Can you work these out from the model? Positions are in its coordinate system, mm. A direction names the side the tool comes from. Give positions to 0.01 mm unless a question says otherwise; leave off trailing zeros. Loops run counter-clockwise (first coordinate to the right, second up) from the corner with the lowest first, then second, coordinate; pieces in that order, holes last. Notation, with made-up numbers: (7, 81.25) - (46, 81.25) arc R15 cw to (46, 92.25) - close; hole circle Ø3 at (46.25, 3). An arc over 180 degrees is marked (long way). Answer as a JSON object with one key per item and string values. Group by question number.
Item 1: Which directions (+Z, -Z, +X, -X, +Y, -Y) give clear straight access to the entire face, cutting with the end or side of a thin tool? Please do faces 1 (the cylindrical face through (-34.07, 6.7, 1.45)), 2 (the flat face through (0, 7.4, 8)), 3 (the flat face through (0, 7.5, 2)).
Item 2: Suppose I cut it at A-A on x = -12.5. Write out the boundary of the cut face in (y, z), and give its area (3 significant figures).
Item 3: Thinking about a two-plate mould opening in X: for faces 4 (the flat face through (0, 3, -4)), 5 (the flat face through (31.5, 6, 2)), 6 (the cylindrical face through (-33.93, 11.9, 6.81)), which applies, pulls with the +X half, pulls with the -X half, needs draft (parallel to the pull), parting line crosses it, or undercut?
Item 4: Suppose I cut it at B-B on y = 1.5. Write out the boundary of the cut face in (x, z), and give its area (3 significant figures).
Item 5: Suppose I cut it at C-C on z = 9.5. Write out the boundary of the cut face in (x, y), and give its area (3 significant figures).
Item 6: Will these pins go through, and if not, where does the flat tip stop? pin 1 (11 mm diameter, centred on x = -16.5, z = -3.5, fed in from +Y); pin 2 (3 mm diameter, centred on x = -3, z = 8, fed in from -Y); pin 3 (1 mm diameter, centred on x = -12, y = 10.5, fed in from -Z).
Item 7: Suppose I cut it at D-D on x = 27. Write out the boundary of the cut face in (y, z), and give its area (3 significant figures).
Item 8: Please list where these lines run through material, in increasing order: L1, parallel to X at y = 1.75, z = 10.25; L2, parallel to Z at x = 18, y = 1.5; L3, parallel to Y at x = 22, z = -4.75.
from build123d import *

# Parameters (mm, degrees)
SKETCH1_W                = 69
SKETCH1_H                = 22
BOSS_EXTRUDE1_DEPTH      = 3
BOSS_EXTRUDE1_DEPTH_BACK = 1
BOSS_EXTRUDE2_DEPTH      = 9.5
CUT_EXTRUDE2_DEPTH       = 63
SKETCH5_W                = 40
SKETCH5_H                = 8.4
CUT_EXTRUDE3_DEPTH       = 6
FILLET5_R                = 2
FILLET6_R                = 1.5


with BuildPart() as part:
    # Sketch1 → Boss-Extrude1 (new body, two sides)
    with BuildSketch(Plane(origin=(0, 0, 0), x_dir=(1, 0, 0), z_dir=(0, 1, 0))) as boss_extrude1_sk:
        Rectangle(SKETCH1_W, SKETCH1_H)
    extrude(amount=BOSS_EXTRUDE1_DEPTH)
    extrude(boss_extrude1_sk.sketch, amount=-BOSS_EXTRUDE1_DEPTH_BACK)

    # Sketch2 → Boss-Extrude2 (add)
    with BuildSketch(Plane(origin=(0, 3, 0), x_dir=(1, 0, 0), z_dir=(0, 1, 0))):
        Polygon((-34.5, -11), (-21.5, -11), (21.5, -11), (34.5, -11), (34.5, -1), (21.5, -1), (-21.5, -1), (-34.5, -1), align=None)
    extrude(amount=BOSS_EXTRUDE2_DEPTH)

    # Sketch4 → Cut-Extrude2 (cut)
    with BuildSketch(Plane(origin=(31.5, 0, 0), x_dir=(0, 0, -1), z_dir=(1, 0, 0))):
        Polygon((-1, 3), (-3.5, 7.5), (-1, 7.5), align=None)
    extrude(amount=-CUT_EXTRUDE2_DEPTH, mode=Mode.SUBTRACT)

    # Sketch5 → Cut-Extrude3 (cut)
    with BuildSketch(Plane.XY.offset(11)):
        with Locations((0, 3.2)):
            Rectangle(SKETCH5_W, SKETCH5_H)
    extrude(amount=-CUT_EXTRUDE3_DEPTH, mode=Mode.SUBTRACT)

    # Fillet5
    fillet5_edges = [part.edges().sort_by_distance(p)[0] for p in [
        (-34.5, 12.5, 6),
        (34.5, 12.5, 6),
    ]]
    fillet(fillet5_edges, radius=FILLET5_R)

    # Fillet6
    fillet6_edges = [part.edges().sort_by_distance(p)[0] for p in [
        (0, 12.5, 1),
        (-34.5, 6.75, 1),
        (34.5, 6.75, 1),
        (33.914213562, 11.914213562, 1),
        (-33.914213562, 11.914213562, 1),
    ]]
    fillet(fillet6_edges, radius=FILLET6_R)


solid = part.part
Worked out:
{
 "1": {"face 1": "-Z, -X, +Y", "face 2": "+Z, -Y", "face 3": "-Z"},
 "2": {"outline": "(-1, -11) - (3, -11) - (3, 1) - (7.5, 3.5) - (7.5, 1) - (11, 1) arc R1.5 ccw to (12.5, 2.5) - (12.5, 11) - (7.4, 11) - (7.4, 5) - (-1, 5) - close", "area": "126 mm2"},
 "3": {"face 4": "needs draft", "face 5": "undercut", "face 6": "pulls with the -X half"},
 "4": {"outline": "(-34.5, -11) - (34.5, -11) - (34.5, 11) - (20, 11) - (20, 5) - (-20, 5) - (-20, 11) - (-34.5, 11) - close", "area": "1,280 mm2"},
 "5": {"outline": "(-34.5, -1) - (-20, -1) - (-20, 7.4) - (20, 7.4) - (20, -1) - (34.5, -1) - (34.5, 10.5) arc R2 ccw to (32.5, 12.5) - (-32.5, 12.5) arc R2 ccw to (-34.5, 10.5) - close", "area": "594 mm2"},
 "6": {"pin 1": "stops at y = 12.41", "pin 2": "stops at y = 7.4", "pin 3": "stops at z = 1"},
 "7": {"outline": "(-1, -11) - (3, -11) - (3, 1) - (7.5, 3.5) - (7.5, 1) - (11, 1) arc R1.5 ccw to (12.5, 2.5) - (12.5, 11) - (-1, 11) - close", "area": "177 mm2"},
 "8": {"L1": "x = -34.5 to -20, 20 to 34.5", "L2": "z = -11 to 5", "L3": "y = -1 to 3"}
}
